Check sheet for the modelled part. Datum: model origin and axes. Units: mm. Face numbers are marked on the shaded views. Give positions to 0.01 mm unless a question says otherwise; leave off trailing zeros. Loops run counter-clockwise (first coordinate to the right, second up) from the corner with the lowest first, then second, coordinate; pieces in that order, holes last. Notation, with made-up numbers: (77, 73) - (118, 73) arc R26 cw to (118, 112) - close; hole circle Ø8 at (-37.75, -19.75). An arc over 180 degrees is marked (long way). Answer in a Markdown table with one row per item. Add a question column.
(1) Sectioned sample at B-B on x = -5.5. Enter the section's corners in (y, z).
(2) Sectioned sample at C-C on y = 2.35. Enter the section's corners in (x, z), then the cut area to 3 significant figures.
(3) Go/stop test with flat-tipped pins: P1, Ø2, axis at x = -24, z = 9.5, coming from the -Y side; P2, Ø1, axis at y = 2, z = 21.5, coming from the -X side. Record where each tip stops, or that it passes through.
(4) Sectioned sample at A-A on z = 0. Enter the section's corners in (x, y).
(5) Draft check along Z on the marked faces 1 and 2. Enter one of: released by +Z, released by -Z, zero draft, split by the parting line, or undercut.
(6) Thickness scan on L1, parallel to X at y = 0.5, z = 0; L2, parallel to X at y = 0.4, z = 4; L3, parallel to Z at x = 28, y = 2.65. Record the ranges inside material, lowest first.
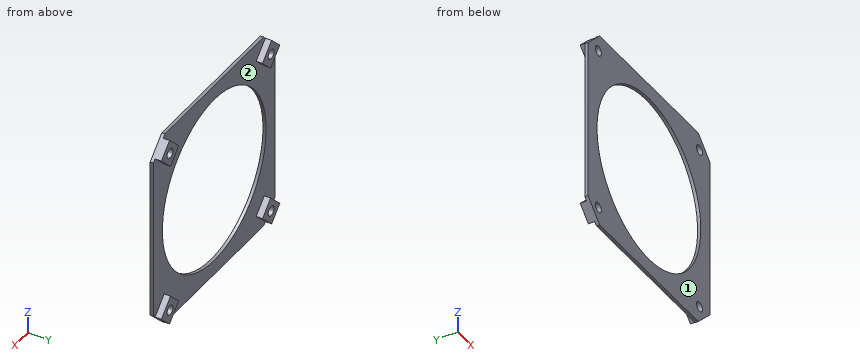
from build123d import *

# Parameters (mm, degrees)
SKETCH1_R            = 27
BOSS_EXTRUDE1_DEPTH  = 1
BOSS_EXTRUDE2_DEPTH  = 2
M3_CLEARANCE_HOLE1_D = 3.1
CIRPATTERN1_COUNT    = 4


with BuildPart() as part:
    # Sketch1 → Boss-Extrude1 (new body)
    with BuildSketch(Plane(origin=(0, 0, 0), x_dir=(1, 0, 0), z_dir=(0, 1, 0))):
        Polygon((31.68, 25.68), (25.68, 31.68), (-25.68, 31.68), (-31.68, 25.68), (-31.68, -25.68), (-25.68, -31.68), (25.68, -31.68), (31.68, -25.68), align=None)
        with Locations(Location((0, 0, 0), (0, 0, 270))):
            Circle(SKETCH1_R, mode=Mode.SUBTRACT)
    extrude(amount=BOSS_EXTRUDE1_DEPTH)

    # Sketch2 → Boss-Extrude2 (add)
    with BuildSketch(Plane(origin=(0, 1, 0), x_dir=(1, 0, 0), z_dir=(0, 1, 0))):
        Polygon((30.801320344, 26.558679656), (26.050064864, 21.807424177), (21.807424177, 26.050064864), (26.558679656, 30.801320344), align=None)
        Polygon((30.801320344, -26.558679656), (26.050064864, -21.807424177), (21.807424177, -26.050064864), (26.558679656, -30.801320344), align=None)
        Polygon((-26.558679656, -30.801320344), (-21.807424177, -26.050064864), (-26.050064864, -21.807424177), (-30.801320344, -26.558679656), align=None)
        Polygon((-30.801320344, 26.558679656), (-26.050064864, 21.807424177), (-21.807424177, 26.050064864), (-26.558679656, 30.801320344), align=None)
    extrude(amount=BOSS_EXTRUDE2_DEPTH)

    # M3 Clearance Hole1 (through all)
    with Locations(Plane(origin=(0, 3, 0), x_dir=(1, 0, 0), z_dir=(0, 1, 0))):
        with Locations((26.30437226, 26.30437226)):
            m3_clearance_hole1 = Hole(M3_CLEARANCE_HOLE1_D / 2)

    # CirPattern1: M3 Clearance Hole1 ×4 about axis
    cirpattern1_axis = Axis((0, 0, 0), (0, 1, 0))
    for i in range(1, CIRPATTERN1_COUNT):
        add(m3_clearance_hole1.rotate(cirpattern1_axis, i * 360 / CIRPATTERN1_COUNT), mode=Mode.SUBTRACT)


solid = part.part
Reply:
| question | item | result |
|---|---|---|
| 1 | outline | (0, -31.68) - (1, -31.68) - (1, -26.43) - (0, -26.43) - close; (0, 26.43) - (1, 26.43) - (1, 31.68) - (0, 31.68) - close |
| 2 | outline | (-30.8, -26.56) - (-26.56, -30.8) - (-21.81, -26.05) - (-26.05, -21.81) - close; (-30.8, 26.56) - (-26.05, 21.81) - (-21.81, 26.05) - (-26.56, 30.8) - close; (21.81, -26.05) - (26.56, -30.8) - (30.8, -26.56) - (26.05, -21.81) - close; (21.81, 26.05) - (26.05, 21.81) - (30.8, 26.56) - (26.56, 30.8) - close; hole circle Ø3.1 at (-26.3, -26.3); hole circle Ø3.1 at (-26.3, 26.3); hole circle Ø3.1 at (26.3, -26.3); hole circle Ø3.1 at (26.3, 26.3) |
| 2 | area | 131 mm^2 |
| 3 | P1 | through |
| 3 | P2 | x = -26.24 |
| 4 | outline | (-31.68, 0) - (-27, 0) - (-27, 1) - (-31.68, 1) - close; (27, 0) - (31.68, 0) - (31.68, 1) - (27, 1) - close |
| 5 | face 1 | zero draft |
| 5 | face 2 | undercut |
| 6 | L1 | -31.68 to -27, 27 to 31.68 |
| 6 | L2 | -31.68 to -26.7, 26.7 to 31.68 |
| 6 | L3 | -29.36 to -23.76, 23.76 to 29.36 |
